Work out the finished part from the listing and answer in its coordinate system (mm). Give positions to 0.01 mm unless a question says otherwise; leave off trailing zeros. Order: outer loops, then holes, each group sorted by start corner. A loop starts at its lowest first (then second) coordinate and runs counter-clockwise, first axis right, second up. Notation, with made-up numbers: (80, -18.75) - (96, -18.75) arc R32 cw to (96, 19.25) - close; hole circle Ø3 at (82.25, 51). An arc over 180 degrees is marked (long way). Put each result on its own line as item: value.
Autodesk Inventor part; units mm, degrees
ref_plane "YZ Plane" through (0, 0, 0) normal (1, 0, 0) x (0, 1, 0)
ref_plane "XZ Plane" through (0, 0, 0) normal (0, 1, 0) x (-1, 0, 0)
ref_plane "XY Plane" through (0, 0, 0) normal (0, 0, 1) x (1, 0, 0)
sketch "Esquisse1" plane through (0, 0, 0) normal (1, 0, 0) x (0, 1, 0)
  line L0 (10, 5) -> (-10, 5)
  line L1 (-10, 5) -> (-10, -5)
  line L2 (-10, -5) -> (10, -5)
  line L3 (10, -5) -> (10, 5)
  line L4 (10, 5) -> (-10, -5) construction
  line L5 (-10, 5) -> (10, -5) construction
  line L6 (11, 6) -> (-11, 6)
  line L7 (-11, 6) -> (-11, -6)
  line L8 (-11, -6) -> (11, -6)
  line L9 (11, -6) -> (11, 6)
  line L10 (11, 6) -> (-11, -6) construction
  line L11 (-11, 6) -> (11, -6) construction
  line L12 (-11, 6) -> (-10, 5) construction
  circle A0 centre (-10.5, 5.5) radius 0.3042
  line L13 (-10, -5) -> (-11, -6) construction
  circle A1 centre (-10.5, -5.5) radius 0.3042
  line L14 (0, 12.1344) -> (0, -11.0693) construction
  line L15 (0, -11.0693) -> (0, -10.4091)
  line L16 (10, 5) -> (11, 6) construction
  line L17 (10, -5) -> (11, -6) construction
  circle A2 centre (10.5, 5.5) radius 0.3042
  circle A3 centre (10.5, -5.5) radius 0.3042
  point P0 (0, 0)
  point P1 (0, 0)
  point P2 (0, 0)
  dimension "d0" = 10
  dimension "d1" = 20
  dimension "d2" = 22
  dimension "d3" = 12
  dimension "d4" = 0.6083
  dimension "d5" = 0.6083
  dimension "d6" = 0.6083
  dimension "d7" = 0.6083
extrude "Extrusion1" add sketch "Esquisse1" along normal blind 1
properties part number "Cadre encoche manette"
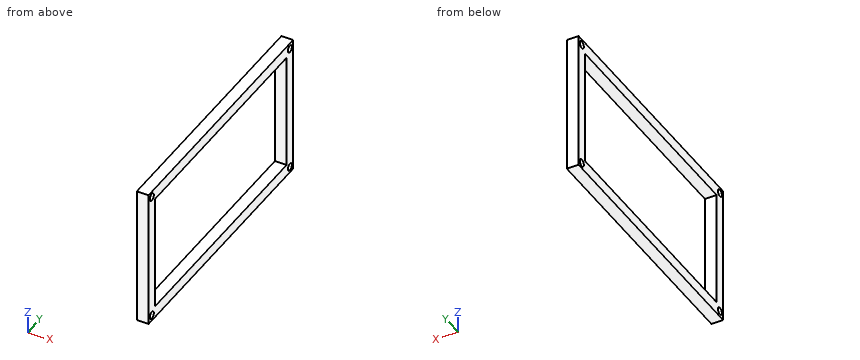
(1) Section A-A, the plane z = -5.5 is taken. Write down the section's boundary in (x, y), then the cut area to 3 significant figures.
Geometry check:
outline: (0, -11) - (1, -11) - (1, -10.8) - (0, -10.8) - close; (0, -10.2) - (1, -10.2) - (1, 10.2) - (0, 10.2) - close; (0, 10.8) - (1, 10.8) - (1, 11) - (0, 11) - close
area: 20.8 mm²
(2) Straight lines are drawn through the part: line 1 (Z direction, x = 0.6, y = 10.5); line 2 (Y direction, x = 0.95, z = 3.5); line 3 (Z direction, x = 0.3, y = 4.5). For each, find the intervals that lie inside material, in ascending order.
Geometry check:
line 1: z = -6 to -5.8, -5.2 to 5.2, 5.8 to 6
line 2: y = -11 to -10, 10 to 11
line 3: z = -6 to -5, 5 to 6
(3) Section C-C, the plane x = 0.85 is taken. Write down the section's boundary in (y, z).
Geometry check:
outline: (-11, -6) - (11, -6) - (11, 6) - (-11, 6) - close; hole circle Ø0.61 at (-10.5, -5.5); hole circle Ø0.61 at (-10.5, 5.5); hole (-10, -5) - (10, -5) - (10, 5) - (-10, 5) - close; hole circle Ø0.61 at (10.5, -5.5); hole circle Ø0.61 at (10.5, 5.5)
(4) Given pin 1 (5 mm diameter, centred on y = -3, z = 3.5, fed in from -X), flat-ended and moving along its own axis, determine where the tip first touches the part or whether it passes through.
Geometry check:
pin 1: stops at x = 0
(5) Section B-B, the plane z = 0 is taken. Write down the section's boundary in (x, y), then the cut area to 3 significant figures.
Geometry check:
outline: (0, -11) - (1, -11) - (1, -10) - (0, -10) - close; (0, 10) - (1, 10) - (1, 11) - (0, 11) - close
area: 2.00 mm²
(6) Section D-D, the plane y = 10.5 is taken. Write down the section's boundary in (x, z).
Geometry check:
outline: (0, -6) - (1, -6) - (1, -5.8) - (0, -5.8) - close; (0, -5.2) - (1, -5.2) - (1, 5.2) - (0, 5.2) - close; (0, 5.8) - (1, 5.8) - (1, 6) - (0, 6) - close
